For this review, take the finished solid that the model builds, in its own axes (mm). A direction names the side the tool comes from. Round coordinates to 2 decimals unless told otherwise and drop trailing zeros. Loops run counter-clockwise (first coordinate to the right, second up) from the corner with the lowest first, then second, coordinate; pieces in that order, holes last.
1. Clearance check with flat-ended pins moving along their axes: pin 1 Ø0.9 at (y, z) = (-5, 6) entering from -X; pin 2 Ø4 at (y, z) = (-3.5, 6.5) entering from +X; pin 3 Ø1 at (x, z) = (3.5, -1.5) entering from -Y. State where each tip first meets the part, or that it passes through.
2. Consider section C-C on y = -5.25. State the section outline as (x, z) points.
3. Consider section B-B on x = 2.39. State the section outline as (y, z) points (3 decimals).
4. Consider section A-A on z = 0.25. State the section outline as (x, y) points, then the cut area to 3 significant figures.
5. Tool access review of faces 5 (the flat face through (2, -5, 9.53)), 6 (the flat face through (0.1, -4, 4)), 7 (the flat face through (4.33, -5, 5)): name each direction out of +Z, -Z, +X, -X, +Y, -Y from which nothing blocks a thin tool from reaching the whole face with its end or side.
6. To check wall thickness, follow line 1 along Y through (x, z) = (4.6, 4.5); line 2 along Z through (x, y) = (1.05, -7); line 3 along X through (y, z) = (-7.5, 1.5). State the ranges of each line that lie inside material, in increasing order.
7. Consider section D-D on z = -4. State the section outline as (x, y) points (3 decimals), then the cut area to 3 significant figures.
8. Draft analysis for pull direction Z (two halves, no side actions). For faces 1 (the flat face through (0.1, -6, 6)), 2 (the flat face through (2, -9.53, 5)), 3 (the flat face through (2, -5, 0)), 4 (the flat face through (0.593, -5.099, 5.138)), state which applies: released by +Z, released by -Z, zero draft, split by the parting line, or undercut.
from build123d import *

# Parameters (mm, degrees)
SKETCH1_W           = 9.53
SKETCH1_H           = 9.53
BASIC_SHAPE_DEPTH   = 4.83
SKETCH3_R           = 2
ADJUSTER_DEPTH      = 0.1
ADJUSTER_SLOT_DEPTH = 1
SKETCH5_R           = 0.25
PINS_DEPTH          = 5
SKETCH6_W           = 0.5
SKETCH6_H           = 7.53
REAR_RELIEF_DEPTH   = 15.53


with BuildPart() as part:
    # Sketch1 → Basic Shape (new body)
    with BuildSketch(Plane(origin=(0, 0, 0), x_dir=(0, 0, 1), z_dir=(1, 0, 0))):
        with Locations((4.765, 4.765)):
            Rectangle(SKETCH1_W, SKETCH1_H)
    extrude(amount=BASIC_SHAPE_DEPTH)

    # Sketch3 → Adjuster (cut)
    with BuildSketch(Plane.YZ):
        with Locations((-4.765, 4.765)):
            Circle(SKETCH3_R)
    extrude(amount=ADJUSTER_DEPTH, mode=Mode.SUBTRACT)

    # Sketch4 → Adjuster Slot (cut)
    with BuildSketch(Plane(origin=(0.1, 0, 0), x_dir=(0, -1, 0), z_dir=(-1, 0, 0))):
        with BuildLine():
            Line((3.749246997, 6.487859784), (6.487859784, 3.749246997))
            ThreePointArc((6.487859784, 3.749246997), (6.179213562, 3.350786438), (5.780753003, 3.042140216))
            Line((5.780753003, 3.042140216), (3.042140216, 5.780753003))
            ThreePointArc((3.042140216, 5.780753003), (3.350786438, 6.179213562), (3.749246997, 6.487859784))
        make_face()
    extrude(amount=-ADJUSTER_SLOT_DEPTH, mode=Mode.SUBTRACT)

    # Sketch5 → Pins (add)
    with BuildSketch(Plane(origin=(0, -19.06, 0), x_dir=(0, -1, 0), z_dir=(0, 0, -1))):
        with Locations((-16.835, -2.39)):
            Circle(SKETCH5_R)
        with Locations((-14.295, -2.39)):
            Circle(SKETCH5_R)
        with Locations((-11.755, -2.39)):
            Circle(SKETCH5_R)
    extrude(amount=PINS_DEPTH)

    # Sketch6 → Rear Relief (cut, through all)
    with BuildSketch(Plane.XY.offset(9.53)):
        with Locations((4.58, -4.765)):
            Rectangle(SKETCH6_W, SKETCH6_H)
    extrude(amount=-REAR_RELIEF_DEPTH, mode=Mode.SUBTRACT)


solid = part.part
Resolved:
1. pin 1: stops at x = 0.1
1. pin 2: stops at x = 4.33
1. pin 3: passes through
2. outline: (0, 0) - (4.33, 0) - (4.33, 9.53) - (0, 9.53) - (0, 6.71) - (0.1, 6.71) - (0.1, 4.99) - (1.1, 4.99) - (1.1, 3.57) - (0.1, 3.57) - (0.1, 2.82) - (0, 2.82) - close
3. outline: (-9.53, 0) - (-7.555, 0) - (-7.555, -5) - (-7.055, -5) - (-7.055, 0) - (-5.015, 0) - (-5.015, -5) - (-4.515, -5) - (-4.515, 0) - (-2.475, 0) - (-2.475, -5) - (-1.975, -5) - (-1.975, 0) - (0, 0) - (0, 9.53) - (-9.53, 9.53) - close
4. outline: (0, -9.53) - (4.83, -9.53) - (4.83, -8.53) - (4.33, -8.53) - (4.33, -1) - (4.83, -1) - (4.83, 0) - (0, 0) - close
4. area: 42.3 mm2
5. face 5: +Z, +X, -X, +Y, -Y
5. face 6: -X
5. face 7: +Z, -Z, +X
6. line 1: y = -9.53 to -8.53, -1 to 0
6. line 2: z = 0 to 9.53
6. line 3: x = 0 to 4.33
7. outline: circle Ø0.5 at (2.39, -7.305); circle Ø0.5 at (2.39, -4.765); circle Ø0.5 at (2.39, -2.225)
7. area: 0.589 mm2
8. face 1: undercut
8. face 2: zero draft
8. face 3: released by -Z
8. face 4: undercut
